Here's how the part is built. I have some questions about the finished solid (model axes, mm). Round coordinates to 2 decimals unless told otherwise and drop trailing zeros. Write each loop counter-clockwise with the first axis right and the second up, starting at its lowest first coordinate (ties: lowest second). Pieces come first, ordered by that corner, then holes. Notation, with made-up numbers: (46.25, -38.5) -> (90.25, -38.5) arc R21 cw to (90.25, -2.5) -> close; hole circle Ø6 at (81, -11). An arc over 180 degrees is marked (long way). Put each result on its own line as item: value. Start each with the question number.
1. Suppose I cut it at A-A (z = 6.5). Please give me the cut outline in (x, y).
2. Suppose I cut it at B-B (x = -134.5). Please give me the cut outline in (y, z), then the cut area to 3 significant figures.
3. I need wall thicknesses on probe 1 along Z at (x, y) = (-127, -14); probe 2 along Y at (x, z) = (-57.5, 3.5); probe 3 along Y at (x, z) = (-78, 2). Which ranges of each line are inside material? Lowest first, please. Write a range as from..to.
4. For pin 1 (12 mm diameter, centred on x = -70.5, z = 16, fed in from +Y); pin 2 (3 mm diameter, centred on x = -44, y = -17, fed in from +Z); pin 3 (6.5 mm diameter, centred on x = -68.5, z = 24, fed in from -Y), each with a flat end and sliding along its axis, tell me the tip position at first contact or that it passes through.
```python
from build123d import *

# Parameters (mm, degrees)
F0_R            = 1.6
F0_W            = 12
F0_H            = 40.5
F0_W_2          = 20
F1_DEPTH        = 2.5
F7_DEPTH        = 3
F9_DEPTH        = 3
F11_DEPTH       = 3
F12_D           = 3.5
F12_CSINK_D     = 6
F12_CSINK_ANGLE = 90
F14_W           = 24
F14_H           = 9
F15_DEPTH       = 32


with BuildPart() as f1:
    # F0 (on Top) → F1 (new body)
    with BuildSketch(Plane.XY):
        Polygon((-139.390603765, 15.5821263526), (-139.390603765, -13.9178736474), (-75.390603765, -13.9178736474), (-75.390603765, 26.5821263526), align=None)
        with BuildLine():
            Line((-75.390603765, -13.9178736474), (-139.390603765, -13.9178736474))
            Line((-139.390603765, -13.9178736474), (-178.390603765, -13.9178736474))
            Line((-178.390603765, -13.9178736474), (-178.390603765, -53.3178736474))
            ThreePointArc((-178.390603765, -53.3178736474), (-177.4360096104, -53.7132794928), (-177.040603765, -54.6678736474))
            ThreePointArc((-177.040603765, -54.6678736474), (-177.4360096104, -55.622467802), (-178.390603765, -56.0178736474))
            Line((-178.390603765, -56.0178736474), (-178.390603765, -60.4178736474))
            ThreePointArc((-178.390603765, -60.4178736474), (-168.1375554378, -56.1709219746), (-163.890603765, -45.9178736474))
            Line((-163.890603765, -45.9178736474), (-163.890603765, -45.4178736474))
            ThreePointArc((-163.890603765, -45.4178736474), (-163.3048173273, -44.003660085), (-161.890603765, -43.4178736474))
            Line((-161.890603765, -43.4178736474), (-139.390603765, -43.4178736474))
            Line((-139.390603765, -43.4178736474), (-75.390603765, -54.4178736474))
            Line((-75.390603765, -54.4178736474), (-63.390603765, -54.4178736474))
            Line((-63.390603765, -54.4178736474), (-63.390603765, -13.9178736474))
            Line((-63.390603765, -13.9178736474), (-75.390603765, -13.9178736474))
        make_face()
        with Locations((-173.390603765, -47.6678736474)):
            Circle(F0_R, mode=Mode.SUBTRACT)
        with BuildLine():
            Line((-178.390603765, -13.9178736474), (-139.390603765, -13.9178736474))
            Line((-139.390603765, -13.9178736474), (-139.390603765, 15.5821263526))
            Line((-139.390603765, 15.5821263526), (-161.890603765, 15.5821263526))
            ThreePointArc((-161.890603765, 15.5821263526), (-163.3048173273, 16.1679127902), (-163.890603765, 17.5821263526))
            Line((-163.890603765, 17.5821263526), (-163.890603765, 18.0821263526))
            Line((-163.890603765, 18.0821263526), (-178.390603765, 18.0821263526))
            Line((-178.390603765, 18.0821263526), (-178.390603765, -13.9178736474))
        make_face()
        with Locations((-69.390603765, 6.3321263526)):
            Rectangle(F0_W, F0_H)
        with BuildLine():
            Line((-178.390603765, -53.3178736474), (-178.390603765, -13.9178736474))
            Line((-178.390603765, -13.9178736474), (-202.390603765, -13.9178736474))
            Line((-202.390603765, -13.9178736474), (-202.390603765, -41.4178736474))
            ThreePointArc((-202.390603765, -41.4178736474), (-201.8048173273, -42.8320872098), (-200.390603765, -43.4178736474))
            Line((-200.390603765, -43.4178736474), (-194.890603765, -43.4178736474))
            ThreePointArc((-194.890603765, -43.4178736474), (-193.4763902026, -44.003660085), (-192.890603765, -45.4178736474))
            Line((-192.890603765, -45.4178736474), (-192.890603765, -45.9178736474))
            ThreePointArc((-192.890603765, -45.9178736474), (-188.6436520922, -56.1709219746), (-178.390603765, -60.4178736474))
            Line((-178.390603765, -60.4178736474), (-178.390603765, -56.0178736474))
            ThreePointArc((-178.390603765, -56.0178736474), (-179.740603765, -54.6678736474), (-178.390603765, -53.3178736474))
        make_face()
        with Locations((-183.390603765, -47.6678736474)):
            Circle(F0_R, mode=Mode.SUBTRACT)
        with BuildLine():
            Line((-202.390603765, -13.9178736474), (-178.390603765, -13.9178736474))
            Line((-178.390603765, -13.9178736474), (-178.390603765, 18.0821263526))
            Line((-178.390603765, 18.0821263526), (-192.890603765, 18.0821263526))
            Line((-192.890603765, 18.0821263526), (-192.890603765, 17.5821263526))
            ThreePointArc((-192.890603765, 17.5821263526), (-193.4763902026, 16.1679127902), (-194.890603765, 15.5821263526))
            Line((-194.890603765, 15.5821263526), (-200.390603765, 15.5821263526))
            ThreePointArc((-200.390603765, 15.5821263526), (-201.8048173273, 14.996339915), (-202.390603765, 13.5821263526))
            Line((-202.390603765, 13.5821263526), (-202.390603765, -13.9178736474))
        make_face()
        with Locations((-53.390603765, 6.3321263526)):
            Rectangle(F0_W_2, F0_H)
        with Locations((-53.390603765, -34.1678736474)):
            Rectangle(F0_W_2, F0_H)
        with BuildLine():
            Line((-178.390603765, 25.4821263526), (-178.390603765, 18.0821263526))
            Line((-178.390603765, 18.0821263526), (-163.890603765, 18.0821263526))
            ThreePointArc((-163.890603765, 18.0821263526), (-168.1375554378, 28.3351746798), (-178.390603765, 32.5821263526))
            Line((-178.390603765, 32.5821263526), (-178.390603765, 28.1821263526))
            ThreePointArc((-178.390603765, 28.1821263526), (-177.4360096104, 27.7867205072), (-177.040603765, 26.8321263526))
            ThreePointArc((-177.040603765, 26.8321263526), (-177.4360096104, 25.877532198), (-178.390603765, 25.4821263526))
        make_face()
        with Locations((-173.390603765, 19.8321263526)):
            Circle(F0_R, mode=Mode.SUBTRACT)
        with BuildLine():
            Line((-192.890603765, 18.0821263526), (-178.390603765, 18.0821263526))
            Line((-178.390603765, 18.0821263526), (-178.390603765, 25.4821263526))
            ThreePointArc((-178.390603765, 25.4821263526), (-179.740603765, 26.8321263526), (-178.390603765, 28.1821263526))
            Line((-178.390603765, 28.1821263526), (-178.390603765, 32.5821263526))
            ThreePointArc((-178.390603765, 32.5821263526), (-188.6436520922, 28.3351746798), (-192.890603765, 18.0821263526))
        make_face()
        with Locations((-183.390603765, 19.8321263526)):
            Circle(F0_R, mode=Mode.SUBTRACT)
        with BuildLine():
            Line((-43.390603765, 26.5821263526), (-43.390603765, -13.9178736474))
            Line((-43.390603765, -13.9178736474), (-23.390603765, -13.9178736474))
            Line((-23.390603765, -13.9178736474), (-23.390603765, 24.5821263526))
            ThreePointArc((-23.390603765, 24.5821263526), (-23.9763902026, 25.996339915), (-25.390603765, 26.5821263526))
            Line((-25.390603765, 26.5821263526), (-43.390603765, 26.5821263526))
        make_face()
        with BuildLine():
            Line((-23.390603765, -13.9178736474), (-43.390603765, -13.9178736474))
            Line((-43.390603765, -13.9178736474), (-43.390603765, -54.4178736474))
            Line((-43.390603765, -54.4178736474), (-25.390603765, -54.4178736474))
            ThreePointArc((-25.390603765, -54.4178736474), (-23.9763902026, -53.8320872098), (-23.390603765, -52.4178736474))
            Line((-23.390603765, -52.4178736474), (-23.390603765, -13.9178736474))
        make_face()
    extrude(amount=F1_DEPTH)

    # F6 (on plane+point) → F7 (join)
    with BuildSketch(Plane.XZ.offset(54.4178736474)):
        with BuildLine():
            Line((-55.390603765, 13), (-55.390603765, 0))
            Line((-55.390603765, 0), (-43.390603765, 0))
            Line((-43.390603765, 0), (-43.390603765, 13))
            Line((-43.390603765, 13), (-45.140603765, 13))
            ThreePointArc((-45.140603765, 13), (-49.390603765, 8.75), (-53.640603765, 13))
            Line((-53.640603765, 13), (-55.390603765, 13))
        make_face()
        with BuildLine():
            ThreePointArc((-43.390603765, 13), (-49.390603765, 19), (-55.390603765, 13))
            Line((-55.390603765, 13), (-53.640603765, 13))
            ThreePointArc((-53.640603765, 13), (-49.390603765, 17.25), (-45.140603765, 13))
            Line((-45.140603765, 13), (-43.390603765, 13))
        make_face()
    extrude(amount=-F7_DEPTH)

    # F8 (on plane+point) → F9 (join)
    with BuildSketch(Plane.XZ.offset(-26.5821263526)):
        with BuildLine():
            Line((-55.390603765, 13), (-55.390603765, 0))
            Line((-55.390603765, 0), (-43.390603765, 0))
            Line((-43.390603765, 0), (-43.390603765, 13))
            Line((-43.390603765, 13), (-45.140603765, 13))
            ThreePointArc((-45.140603765, 13), (-49.390603765, 8.75), (-53.640603765, 13))
            Line((-53.640603765, 13), (-55.390603765, 13))
        make_face()
        with BuildLine():
            ThreePointArc((-43.390603765, 13), (-49.390603765, 19), (-55.390603765, 13))
            Line((-55.390603765, 13), (-53.640603765, 13))
            ThreePointArc((-53.640603765, 13), (-49.390603765, 17.25), (-45.140603765, 13))
            Line((-45.140603765, 13), (-43.390603765, 13))
        make_face()
    extrude(amount=F9_DEPTH)

    # F10 (on plane+point) → F11 (join)
    with BuildSketch(Plane.XZ.offset(-16.5821263526)):
        with BuildLine():
            Line((-79.390603765, 22.5), (-79.390603765, 0))
            Line((-79.390603765, 0), (-58.390603765, 0))
            Line((-58.390603765, 0), (-58.390603765, 22.5))
            Line((-58.390603765, 22.5), (-64.6479630778, 22.5))
            ThreePointArc((-64.6479630778, 22.5), (-64.4554102465, 21.7609589043), (-64.390603765, 21))
            ThreePointArc((-64.390603765, 21), (-65.7086232496, 17.8180194847), (-68.890603765, 16.5))
            ThreePointArc((-68.890603765, 16.5), (-72.0725842803, 17.8180194847), (-73.390603765, 21))
            ThreePointArc((-73.390603765, 21), (-73.3257972834, 21.7609589043), (-73.1332444521, 22.5))
            Line((-73.1332444521, 22.5), (-79.390603765, 22.5))
        make_face()
        with BuildLine():
            ThreePointArc((-68.890603765, 33), (-76.3152249674, 29.9246212025), (-79.390603765, 22.5))
            Line((-79.390603765, 22.5), (-73.1332444521, 22.5))
            ThreePointArc((-73.1332444521, 22.5), (-72.696981914, 23.4003094356), (-72.0725842803, 24.1819805153))
            ThreePointArc((-72.0725842803, 24.1819805153), (-70.6126792106, 25.1574578963), (-68.890603765, 25.5))
            Line((-68.890603765, 25.5), (-68.890603765, 33))
        make_face()
        with BuildLine():
            Line((-64.6479630778, 22.5), (-58.390603765, 22.5))
            ThreePointArc((-58.390603765, 22.5), (-61.4659825625, 29.9246212025), (-68.890603765, 33))
            Line((-68.890603765, 33), (-68.890603765, 25.5))
            ThreePointArc((-68.890603765, 25.5), (-66.2925275536, 24.6742346142), (-64.6479630778, 22.5))
        make_face()
    extrude(amount=F11_DEPTH)

    # F12 (through all)
    with Locations(Plane(origin=(0, 16.5821263526, 0), x_dir=(1, 0, 0), z_dir=(0, 1, 0))):
        with Locations((-74.901011405, -27.0104076401), (-62.8801961249, -27.0104076401), (-62.8801961249, -14.9895923599), (-74.901011405, -14.9895923599)):
            CounterSinkHole(F12_D / 2, F12_CSINK_D / 2, counter_sink_angle=F12_CSINK_ANGLE)

    # F14 (on plane+point) → F15 (join)
    with BuildSketch(Plane.XZ.offset(15.4178736474)):
        with Locations((-67.390603765, 4.5)):
            Rectangle(F14_W, F14_H)
    extrude(amount=-F15_DEPTH)


solid = f1.part
```
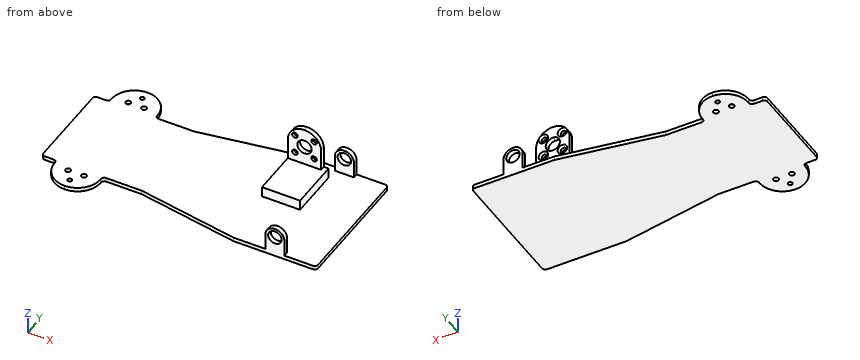
Verdict:
1. outline: (-79.39, -15.42) -> (-55.39, -15.42) -> (-55.39, 16.58) -> (-79.39, 16.58) -> close; (-55.39, -54.42) -> (-43.39, -54.42) -> (-43.39, -51.42) -> (-55.39, -51.42) -> close; (-55.39, 23.58) -> (-43.39, 23.58) -> (-43.39, 26.58) -> (-55.39, 26.58) -> close
2. outline: (-44.26, 0) -> (16.42, 0) -> (16.42, 2.5) -> (-44.26, 2.5) -> close
2. area: 152 mm^2
3. probe 1: z = 0..2.5
3. probe 2: y = -15.42..16.58
3. probe 3: y = -53.97..26.13
4. pin 1: stops at y = 16.58
4. pin 2: stops at z = 2.5
4. pin 3: stops at y = 13.58
